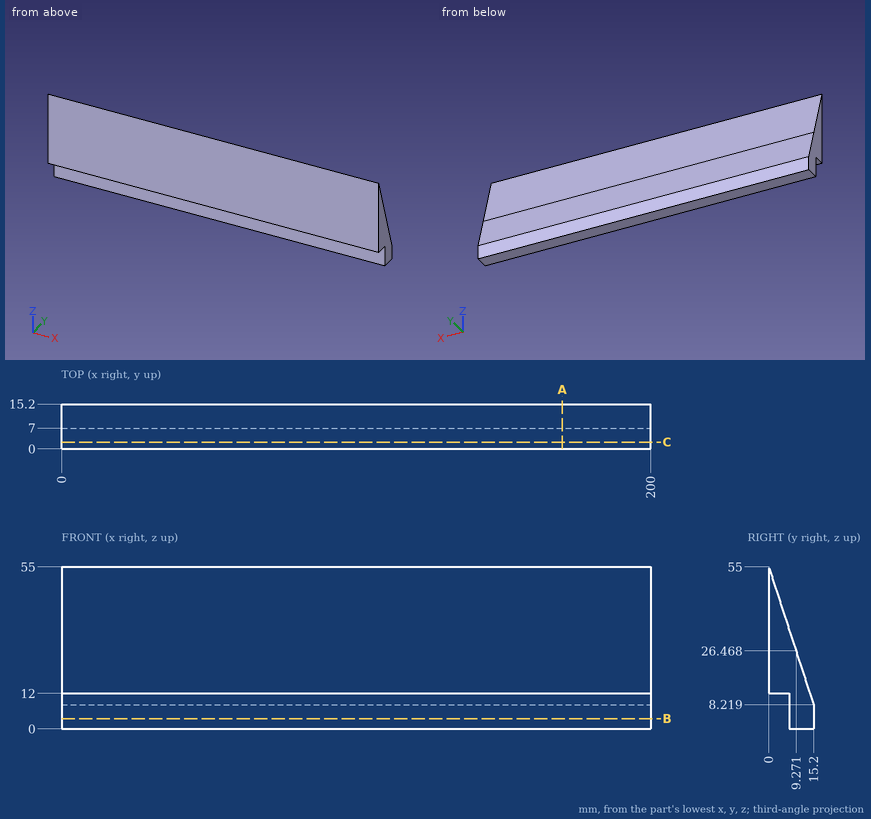
Part print with two shaded views. Sizes in mm from the minimum x, y, z corner. Give positions to 0.01 mm unless a question says otherwise; leave off trailing zeros. Write each loop counter-clockwise with the first axis right and the second up, starting at its lowest first coordinate (ties: lowest second). Pieces come first, ordered by that corner, then holes.
1) Cut at A-A on x = 170. Write the cut outline in (y, z).
Resolved:
outline: (0, 12) - (7, 12) - (7, 0) - (15.2, 0) - (15.2, 8.22) - (0, 55) - close
2) Pin check, flat tips, straight feed: pin 1 (2 mm diameter, centred on x = 165.5, y = 3.5, fed in from -Z); pin 2 (8 mm diameter, centred on x = 107, z = 20.5, fed in from +Y); pin 3 (10 mm diameter, centred on x = 96.5, z = 48, fed in from +Y); pin 4 (4 mm diameter, centred on x = 42, z = 44, fed in from -Y). Stop position of each tip, or through.
Resolved:
pin 1: stops at z = 12
pin 2: stops at y = 12.51
pin 3: stops at y = 3.9
pin 4: stops at y = 0
3) Cut at C-C on y = 2.25. Write the cut outline in (x, z) (1 decimal).
Resolved:
outline: (0, 12) - (200, 12) - (200, 48.1) - (0, 48.1) - close
4) Cut at B-B on z = 3.5. Write the cut outline in (x, y).
Resolved:
outline: (0, 7) - (200, 7) - (200, 15.2) - (0, 15.2) - close
5) Probe L1, parallel to Y at x = 106.5, z = 7; L2, parallel to Y at x = 59, z = 26.5. List the from-to ranges inside material, lowest first.
Resolved:
L1: y = 7 to 15.2
L2: y = 0 to 9.26
